```python
from build123d import *

# Parameters (mm, degrees)
BOSS_EXTRUDE1_DEPTH = 38
SKETCH2_R           = 1.5
CUT_EXTRUDE1_DEPTH  = 11


with BuildPart() as part:
    # Sketch1 → Boss-Extrude1 (new body)
    with BuildSketch(Plane.XY):
        with BuildLine():
            Line((10.65, -8), (11.4, -8))
            Line((11.4, -8), (11.4, 8))
            Line((11.4, 8), (10.65, 8))
            Line((10.65, 8), (10.65, 0.8))
            Line((10.65, 0.8), (-10.65, 0.8))
            Line((-10.65, 0.8), (-10.65, 8))
            Line((-10.65, 8), (-11.4, 8))
            Line((-11.4, 8), (-11.4, -8))
            Line((-11.4, -8), (-10.65, -8))
            Line((-10.65, -8), (-10.65, -0.8))
            Line((-10.65, -0.8), (-6.99, -0.8))
            Line((-6.99, -0.8), (-6.99, -8))
            Line((-6.99, -8), (-6.24, -8))
            Line((-6.24, -8), (-6.24, -0.8))
            Line((-6.24, -0.8), (-2.58, -0.8))
            Line((-2.58, -0.8), (-2.58, -8))
            Line((-2.58, -8), (-1.83, -8))
            Line((-1.83, -8), (-1.83, -3.8))
            Line((-1.83, -3.8), (-1.83, -0.8))
            Line((-1.83, -0.8), (-0.538516481, -0.8))
            ThreePointArc((-0.538516481, -0.8), (0, -0.7), (0.538516481, -0.8))
            Line((0.538516481, -0.8), (1.83, -0.8))
            Line((1.83, -0.8), (1.83, -3.8))
            Line((1.83, -3.8), (1.83, -8))
            Line((1.83, -8), (2.58, -8))
            Line((2.58, -8), (2.58, -0.8))
            Line((2.58, -0.8), (6.24, -0.8))
            Line((6.24, -0.8), (6.24, -8))
            Line((6.24, -8), (6.99, -8))
            Line((6.99, -8), (6.99, -0.8))
            Line((6.99, -0.8), (10.65, -0.8))
            Line((10.65, -0.8), (10.65, -8))
        make_face()
        with BuildLine():
            Line((-1.83, -0.8), (-1.83, -3.8))
            Line((-1.83, -3.8), (-1.08, -3.8))
            Line((-1.08, -3.8), (-1.08, -3.240961094))
            ThreePointArc((-1.08, -3.240961094), (-1.46440147, -1.87514875), (-0.538516481, -0.8))
            Line((-0.538516481, -0.8), (-1.83, -0.8))
        make_face()
        with BuildLine():
            Line((-0.538516481, -0.8), (0.538516481, -0.8))
            ThreePointArc((0.538516481, -0.8), (0, -0.7), (-0.538516481, -0.8))
        make_face()
        with BuildLine():
            Line((1.08, -3.8), (1.83, -3.8))
            Line((1.83, -3.8), (1.83, -0.8))
            Line((1.83, -0.8), (0.538516481, -0.8))
            ThreePointArc((0.538516481, -0.8), (1.46440147, -1.87514875), (1.08, -3.240961094))
            Line((1.08, -3.240961094), (1.08, -3.8))
        make_face()
    extrude(amount=BOSS_EXTRUDE1_DEPTH)

    # Sketch2 → Cut-Extrude1 (cut)
    with BuildSketch(Plane(origin=(0, 0.8, 0), x_dir=(1, 0, 0), z_dir=(0, 1, 0))):
        with Locations(Location((0, -21.5, 0), (0, 0, 180))):
            Circle(SKETCH2_R)
    extrude(amount=-CUT_EXTRUDE1_DEPTH, mode=Mode.SUBTRACT)


solid = part.part
```
Build history of the part. All positions in model axes, mm. A direction names the side the tool comes from. Coordinates: 2 decimals unless noted, no trailing zeros. Order: outer loops, then holes, each group sorted by start corner. A loop starts at its lowest first (then second) coordinate and runs counter-clockwise, first axis right, second up. Notation, with made-up numbers: (-31.5, 52) -> (-12.5, 52) arc R15 cw to (-12.5, 64) -> close; hole circle Ø6 at (-16, 77.5). An arc over 180 degrees is marked (long way). Answer in a Markdown table with one row per item. Add a question column.
Q1. Band-saw the part on A-A, the plane x = 0. List the corners of the cut face in (y, z).
Q2. Band-saw the part on C-C, the plane y = 3.25. List the corners of the cut face in (x, z), then the cut area to 3 significant figures.
Q3. Which spindle directions (+Z, -Z, +X, -X, +Y, -Y) get a long thin tool onto all of the face, cutting with end or side? Do faces 4 (the face through (-1.47, -1.9, 10.6)), 5 (the face through (-10.65, 4, 19)), 6 (the face through (6.24, -4, 19)). Say none if no direction does.
Q4. Wall check: line 1 along X through (y, z) = (-2, 21.5); line 2 along X through (y, z) = (-4.75, 33); line 3 along X through (y, z) = (2.25, 13.5). Give the ranges that are in metal, low to high. Write a range as [from, to].
Q5. Band-saw the part on B-B, the plane y = -6.5. List the corners of the cut face in (x, z).
Q6. Drop flat-ended pins along their axis: pin 1 (0.6 mm diameter, centred on x = 1.5, z = 11.5, fed in from -Y); pin 2 (6.5 mm diameter, centred on x = -1.5, z = 10, fed in from +Y); pin 3 (0.9 mm diameter, centred on x = 0, z = 28.5, fed in from -Y). Give the stop position or say it passes through.
Q7. Mould opens along X. For faces 1 (the face through (-11.4, 0, 19)), 2 (the face through (11.4, 0, 19)), 3 (the face through (2.58, -4, 19)) say: +X half, -X half, draft (parallel to the pull), parting line (faces both ways), or undercut.
Answers follow:
| question | item | result |
|---|---|---|
| 1 | outline | (-0.8, 0) -> (0.8, 0) -> (0.8, 20) -> (-0.8, 20) -> close; (-0.8, 23) -> (0.8, 23) -> (0.8, 38) -> (-0.8, 38) -> close |
| 2 | outline | (-11.4, 0) -> (-10.65, 0) -> (-10.65, 38) -> (-11.4, 38) -> close; (10.65, 0) -> (11.4, 0) -> (11.4, 38) -> (10.65, 38) -> close |
| 2 | area | 57.0 mm^2 |
| 3 | face 4 | +Z, -Z |
| 3 | face 5 | +Z, -Z, +Y |
| 3 | face 6 | +Z, -Z, -Y |
| 4 | line 1 | [-11.4, -10.65], [-6.99, -6.24], [-2.58, -1.5], [1.5, 2.58], [6.24, 6.99], [10.65, 11.4] |
| 4 | line 2 | [-11.4, -10.65], [-6.99, -6.24], [-2.58, -1.83], [1.83, 2.58], [6.24, 6.99], [10.65, 11.4] |
| 4 | line 3 | [-11.4, -10.65], [10.65, 11.4] |
| 5 | outline | (-11.4, 0) -> (-10.65, 0) -> (-10.65, 38) -> (-11.4, 38) -> close; (-6.99, 0) -> (-6.24, 0) -> (-6.24, 38) -> (-6.99, 38) -> close; (-2.58, 0) -> (-1.83, 0) -> (-1.83, 38) -> (-2.58, 38) -> close; (1.83, 0) -> (2.58, 0) -> (2.58, 38) -> (1.83, 38) -> close; (6.24, 0) -> (6.99, 0) -> (6.99, 38) -> (6.24, 38) -> close; (10.65, 0) -> (11.4, 0) -> (11.4, 38) -> (10.65, 38) -> close |
| 6 | pin 1 | y = -3.8 |
| 6 | pin 2 | y = 0.8 |
| 6 | pin 3 | y = -0.8 |
| 7 | face 1 | -X half |
| 7 | face 2 | +X half |
| 7 | face 3 | undercut |
